```python
from build123d import *

# Parameters (mm, degrees)
BOSS_EXTRUDE1_DEPTH = 7
FILLET1_R           = 2
SKETCH3_R           = 1.5
SKETCH3_R_2         = 1.1
BOSS_EXTRUDE2_DEPTH = 4
SKETCH4_R           = 1.5
SKETCH4_R_2         = 1.1
SKETCH4_W           = 4.5
SKETCH4_H           = 1.5
BOSS_EXTRUDE3_DEPTH = 4


with BuildPart() as part:
    # Sketch1 → Boss-Extrude1 (new body)
    with BuildSketch(Plane(origin=(0, 0, 0), x_dir=(1, 0, 0), z_dir=(0, 1, 0))):
        with BuildLine():
            Line((10, -9), (-10, -9))
            ThreePointArc((-10, -9), (-11.414213562, -8.414213562), (-12, -7))
            Line((-12, -7), (-12, 7))
            ThreePointArc((-12, 7), (-11.414213562, 8.414213562), (-10, 9))
            Line((-10, 9), (10, 9))
            ThreePointArc((10, 9), (11.414213562, 8.414213562), (12, 7))
            Line((12, 7), (12, -7))
            ThreePointArc((12, -7), (11.414213562, -8.414213562), (10, -9))
        make_face()
    extrude(amount=BOSS_EXTRUDE1_DEPTH)

    # Fillet1
    fillet1_edges = [part.edges().sort_by_distance(p)[0] for p in [
        (12, 0, 0),
        (11.414213562, 0, 8.414213562),
        (0, 0, 9),
        (-11.414213562, 0, 8.414213562),
        (11.414213562, 7, 8.414213562),
        (12, 7, 0),
        (11.414213562, 7, -8.414213562),
        (0, 7, -9),
        (-11.414213562, 7, -8.414213562),
        (-12, 7, 0),
        (-11.414213562, 7, 8.414213562),
        (-12, 0, 0),
        (0, 7, 9),
        (-11.414213562, 0, -8.414213562),
        (0, 0, -9),
        (11.414213562, 0, -8.414213562),
    ]]
    fillet(fillet1_edges, radius=FILLET1_R)

    # Sketch3 → Boss-Extrude2 (add)
    with BuildSketch(Plane.ZY.offset(12)):
        with Locations((7, 3.5)):
            Circle(SKETCH3_R)
        with Locations((7, 3.5)):
            Circle(SKETCH3_R_2, mode=Mode.SUBTRACT)
        with Locations((0, 3.5)):
            Circle(SKETCH3_R)
        with Locations((0, 3.5)):
            Circle(SKETCH3_R_2, mode=Mode.SUBTRACT)
        with Locations((-7, 3.5)):
            Circle(SKETCH3_R)
        with Locations((-7, 3.5)):
            Circle(SKETCH3_R_2, mode=Mode.SUBTRACT)
    extrude(amount=BOSS_EXTRUDE2_DEPTH)

    # Sketch4 → Boss-Extrude3 (add)
    with BuildSketch(Plane(origin=(12, 0, 0), x_dir=(0, 0, -1), z_dir=(1, 0, 0))):
        with Locations((-4.680368176, 3.5)):
            Circle(SKETCH4_R)
        with Locations((-4.680368176, 3.5)):
            Circle(SKETCH4_R_2, mode=Mode.SUBTRACT)
        with Locations((0, 3.5)):
            Circle(SKETCH4_R)
        with Locations((0, 3.5)):
            Circle(SKETCH4_R_2, mode=Mode.SUBTRACT)
        with Locations((5.830286219, 3.5)):
            Rectangle(SKETCH4_W, SKETCH4_H)
    extrude(amount=BOSS_EXTRUDE3_DEPTH)


solid = part.part
```
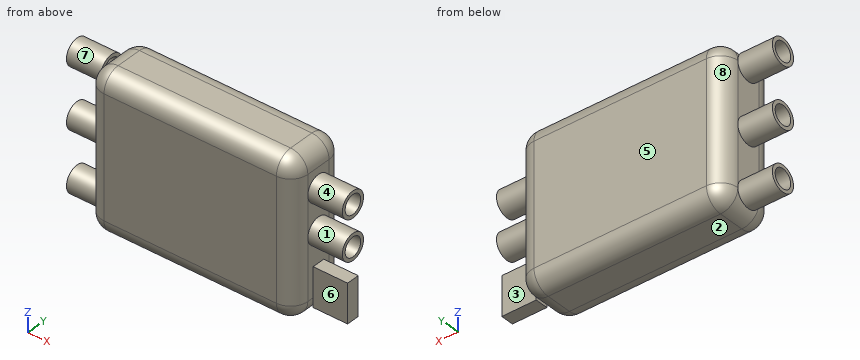
The model under review builds one solid part; all positions refer to its coordinate system, in mm. Face numbers are marked on the shaded views. A direction names the side the tool comes from. Give positions to 0.01 mm unless a question says otherwise; leave off trailing zeros. Write each loop counter-clockwise with the first axis right and the second up, starting at its lowest first coordinate (ties: lowest second). Pieces come first, ordered by that corner, then holes. Notation, with made-up numbers: M 81,43.5 L 101,43.5 A14 cw 101,49.5 Z; hole C -38,72.25 d3. An arc over 180 degrees is marked long. Write item = value, one per line. Start each with the question number.
Q1. We need section A-A (x = 7). State the section outline as (y, z) points, plus the area to 3 significant figures.
Q2. For line 1 (Y direction, x = 13.95, z = 0); line 2 (X direction, y = 4.5, z = 4.75); line 3 (Y direction, x = 12.5, z = 0.5), list the stretches that pass through material, from the lowest coordinate up.
Q3. Mouldability with a two-part tool opening along Z and no side actions: class the marked faces 1, 2 and 3 as released by +Z, released by -Z, zero draft, split by the parting line, or undercut.
Q4. Clearance check with flat-ended pins moving along their axes: pin 1 (0.6 mm diameter, centred on y = 4, z = 6.5, fed in from -X); pin 2 (1.2 mm diameter, centred on x = 14, z = -6.5, fed in from +Y); pin 3 (1.5 mm diameter, centred on x = 0, y = 1, fed in from -Z). State where each tip first meets the part, or that it passes through.
Q5. Machinability: for the marked faces 4, 5, 6, 7 and 8, which of the approach directions +Z, -Z, +X, -X, +Y, -Y give a long, thin tool a straight path to every point of the face, cutting with its end or side? Answer none if there is none.
Q6. We need section B-B (z = 2.25). State the section outline as (x, y) points.
Q7. We need section C-C (y = 3.5). Give the number of separate pieces and of enclosed holes in the cut face, plus the area to 3 significant figures.
Result set:
q1.outline = M 0,-7 A2 ccw 2,-9 L 5,-9 A2 ccw 7,-7 L 7,7 A2 ccw 5,9 L 2,9 A2 ccw 0,7 Z
q1.area = 123 mm2
q2.line_1 = 2 to 2.4, 4.6 to 5
q2.line_2 = -12 to 12
q2.line_3 = 2.09 to 2.52, 4.48 to 4.91
q3.face_1 = undercut
q3.face_2 = released by -Z
q3.face_3 = zero draft
q4.pin_1 = -12
q4.pin_2 = 4.25
q4.pin_3 = -8.98
q5.face_4 = +X
q5.face_5 = +Z, -Z, +X, -X, +Y
q5.face_6 = -Z, +X, -Y
q5.face_7 = -X
q5.face_8 = +Z, -Z, -X, +Y
q6.outline = M -12,2 A2 ccw -10,0 L 10,0 A2 ccw 12,2 L 12,5 A2 ccw 10,7 L -10,7 A2 ccw -12,5 Z
q7.separate_pieces = 3
q7.enclosed_holes = 0
q7.area = 463 mm2
